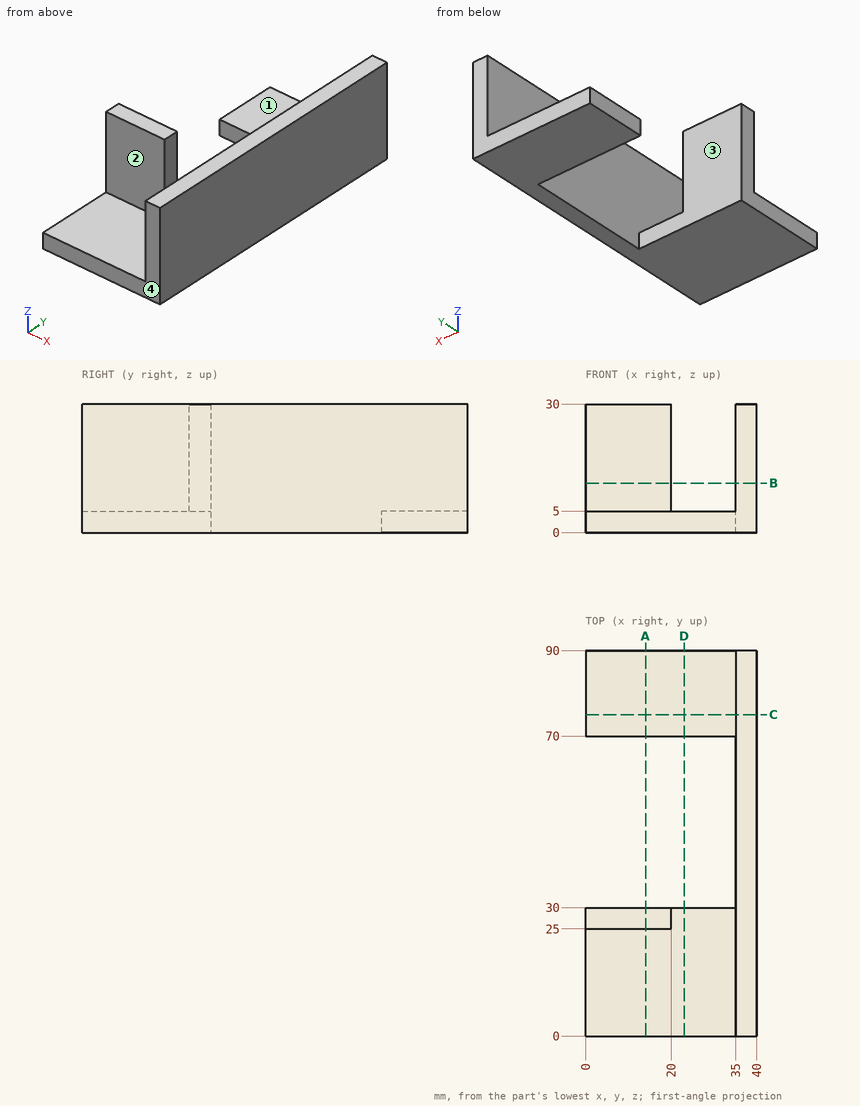
Check sheet for the drawn part. Datum: minimum x, y, z corner. Units: mm. A direction names the side the tool comes from. Round coordinates to 2 decimals unless told otherwise and drop trailing zeros. Order: outer loops, then holes, each group sorted by start corner. A loop starts at its lowest first (then second) coordinate and runs counter-clockwise, first axis right, second up. Notation, with made-up numbers: (43.5, -33.5) -> (86.5, -33.5) arc R22 ccw to (86.5, 0.5) -> close; hole circle Ø3 at (76, -36). An arc over 180 degrees is marked (long way). Put each result on its own line as item: value.
1) Set-up check for the marked faces 1, 2, 3 and 4: record each of +Z, -Z, +X, -X, +Y, -Y from which the full face is reachable in a straight line by a thin tool's end or side.
Final values:
face 1: +Z, -X, +Y
face 2: +Z, -X, -Y
face 3: +Z, -Z, -X
face 4: +Z, -Z, +X, -X, -Y
2) Section check C-C (y = 75). Record the cut outline in (x, z).
Final values:
outline: (0, 0) -> (40, 0) -> (40, 30) -> (35, 30) -> (35, 5) -> (0, 5) -> close
3) Section check A-A (x = 14). Record the cut outline in (y, z), then the cut area to 3 significant figures.
Final values:
outline: (0, 0) -> (30, 0) -> (30, 30) -> (25, 30) -> (25, 5) -> (0, 5) -> close; (70, 0) -> (90, 0) -> (90, 5) -> (70, 5) -> close
area: 375 mm^2
4) Section check B-B (z = 11.5). Record the cut outline in (x, y).
Final values:
outline: (0, 25) -> (20, 25) -> (20, 30) -> (0, 30) -> close; (35, 0) -> (40, 0) -> (40, 90) -> (35, 90) -> close
5) Depth check by flat-ended pin: pin 1 (10 mm diameter, centred on y = 47, z = 22.5, fed in from -X); pin 2 (12 mm diameter, centred on x = 18, y = 37.5, fed in from +Z); pin 3 (6 mm diameter, centred on x = 21, y = 77.5, fed in from +Z); pin 4 (16 mm diameter, centred on x = 8.5, z = 17.5, fed in from -Y). Enter the tip coordinate at first touch or a pass-through.
Final values:
pin 1: stops at x = 35
pin 2: passes through
pin 3: stops at z = 5
pin 4: stops at y = 25
6) Section check D-D (x = 23). Record the cut outline in (y, z).
Final values:
outline: (0, 0) -> (30, 0) -> (30, 5) -> (0, 5) -> close; (70, 0) -> (90, 0) -> (90, 5) -> (70, 5) -> close
7) Material ranges on line 1 (Y direction, x = 32, z = 3.25); line 2 (Y direction, x = 19.5, z = 14.75); line 3 (X direction, y = 19.5, z = 12.5), recorded low to high.
Final values:
line 1: y = 0 to 30, 70 to 90
line 2: y = 25 to 30
line 3: x = 35 to 40
